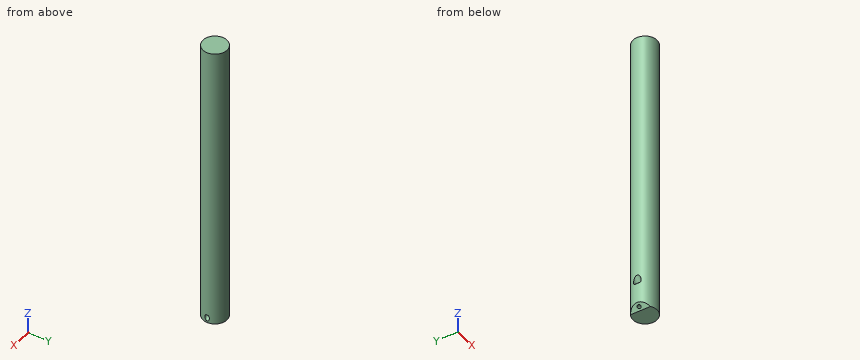
```python
from build123d import *

# Parameters (mm, degrees)
SKETCH1_R                   = 12.7
EXTRUDE1_DEPTH              = 304.8
SKETCH4_R                   = 2.38125
EXTRUDE2_DEPTH              = 306.328708116
EXTRUDE2_DEPTH_BACK         = 306.328708116
SKETCH6_W                   = 20.167016722
SKETCH6_H                   = 37.330359398
EXTRUDE3_DEPTH              = 63.5
F_10_24_TAPPED_HOLE1_REACH  = 305.254
F_10_24_TAPPED_HOLE1_BORE_R = 1.89865
SKETCH10_R                  = 3.96875
EXTRUDE4_DEPTH              = 288.166292049


with BuildPart() as part:
    # Sketch1 → Extrude1 (new body)
    with BuildSketch(Plane.XY):
        with Locations(Location((0, 0, 0), (0, 0, 180))):
            Circle(SKETCH1_R)
    extrude(amount=EXTRUDE1_DEPTH)

    # Sketch4 → Extrude2 (cut, two sides)
    with BuildSketch(Plane(origin=(0, 0, 0), x_dir=(0.7071067811865462, 0, 0.7071067811865488), z_dir=(-0.7071067811865488, 0, 0.7071067811865462))) as extrude2_sk:
        with Locations((12.7, 0)):
            Circle(SKETCH4_R)
    extrude(amount=EXTRUDE2_DEPTH, mode=Mode.SUBTRACT)
    extrude(extrude2_sk.sketch, amount=-EXTRUDE2_DEPTH_BACK, mode=Mode.SUBTRACT)

    # Sketch6 → Extrude3 (cut)
    with BuildSketch(Plane(origin=(-3.592102448, 0, -3.592102448), x_dir=(-0.7071067811865512, 0, 0.7071067811865438), z_dir=(-0.7071067811865438, 0, -0.7071067811865512))):
        with Locations((5.167476491, 0)):
            Rectangle(SKETCH6_W, SKETCH6_H)
    extrude(amount=EXTRUDE3_DEPTH, mode=Mode.SUBTRACT)

    # #10-24 Tapped Hole1 bore (on position points) → #10-24 Tapped Hole1 (cut, up to next)
    with BuildSketch(Plane(origin=(-9.846920352, -0.244294465, 2.662715455), x_dir=(-0.707106781187, 0, 0.707106781187), z_dir=(-0.707106781187, 0, -0.707106781187)), mode=Mode.PRIVATE) as f_10_24_tapped_hole1_sk1:
        Circle(F_10_24_TAPPED_HOLE1_BORE_R)
    f_10_24_tapped_hole1_tool1 = extrude(f_10_24_tapped_hole1_sk1.sketch, amount=-F_10_24_TAPPED_HOLE1_REACH, mode=Mode.PRIVATE) & part.part
    add(f_10_24_tapped_hole1_tool1.solids().sort_by_distance((-9.84692, -0.244294, 2.662715))[0], mode=Mode.SUBTRACT)

    # Sketch10 → Extrude4 (cut, through all)
    with BuildSketch(Plane(origin=(-19.756563466, 0, 19.756563466), x_dir=(0.7071067811865462, 0, 0.7071067811865488), z_dir=(-0.7071067811865488, 0, 0.7071067811865462))):
        with Locations((12.7, 0)):
            Circle(SKETCH10_R)
    extrude(amount=EXTRUDE4_DEPTH, mode=Mode.SUBTRACT)


solid = part.part
```
Geometry check sheet. Reference: the model listing, model coordinates, mm. Coordinates: 2 decimals unless noted, no trailing zeros. Order: outer loops, then holes, each group sorted by start corner. A loop starts at its lowest first (then second) coordinate and runs counter-clockwise, first axis right, second up. Notation, with made-up numbers: M 65,-16 L 90,-16 A22 ccw 90,-4 Z; hole C 54,-29.5 d7. An arc over 180 degrees is marked long. Answer as a JSON object with one key per item and string values.
Q1. Cross-section at B-B on x = -3. Give the number of separate pieces and of enclosed holes in the cut face, and give its area (3 significant figures).
Results are:
{"separate pieces": "1", "enclosed holes": "2", "area": "7,480 mm²"}
Q2. Cross-section at A-A on z = 248.5. Record the cut outline in (x, y), and give its area (3 significant figures).
Results are:
{"outline": "C 0,0 d25.4", "area": "507 mm²"}
Q3. Scan lines: line 1 (Y direction, x = 0.75, z = 88); line 2 (Z direction, x = 8.5, y = -0.5); line 3 (Z direction, x = -11.25, y = 1.5). Record each from-to range of solid material in increasing order.
Results are:
{"line 1": "y = -12.68 to 12.68", "line 2": "z = 0 to 6.17, 12.75 to 304.8", "line 3": "z = 4.07 to 26.6, 34.41 to 304.8"}
Q4. Depth check by flat-ended pin: pin 1 Ø1 at (x, z) = (-9.5, 159) entering from -Y; pin 2 Ø12 at (y, z) = (6, 107) entering from +X; pin 3 Ø5 at (x, z) = (-6, 204) entering from -Y; pin 4 Ø3 at (x, z) = (-2, 162.5) entering from -Y. Enter the tip coordinate at first touch or a pass-through.
Results are:
{"pin 1": "stops at y = -8.96", "pin 2": "stops at x = 12.7", "pin 3": "stops at y = -12.21", "pin 4": "stops at y = -12.69"}
